```python
from build123d import *

# Parameters (mm, degrees)
BOSS_EXTRUDE1_DEPTH    = 201
CUT_EXTRUDE1_START     = -40
CUT_EXTRUDE1_OUTLINE_W = 106
CUT_EXTRUDE1_OUTLINE_H = 171
CUT_EXTRUDE1_DEPTH     = 40
SKETCH3_R              = 7.5
BOSS_EXTRUDE2_DEPTH    = 171
SKETCH4_W              = 15
SKETCH4_H              = 171
CUT_EXTRUDE2_DEPTH     = 12.5


# Read off the part's stored shape, not the designer's step: Cut-Extrude1
with BuildPart() as part:
    # Sketch1 → Boss-Extrude1 (new body)
    with BuildSketch(Plane(origin=(0, 0, 0), x_dir=(1, 0, 0), z_dir=(0, 1, 0))):
        with BuildLine():
            Line((-100, 20), (0, 20))
            ThreePointArc((0, 20), (20, 0), (0, -20))
            Line((0, -20), (-100, -20))
            Line((-100, -20), (-100, 20))
        make_face()
    extrude(amount=BOSS_EXTRUDE1_DEPTH)

    # Cut-Extrude1 outline → Cut-Extrude1 (cut)
    with BuildSketch(Plane.XY.offset(20).offset(CUT_EXTRUDE1_START)):
        with Locations((-32, 100.5)):
            Rectangle(CUT_EXTRUDE1_OUTLINE_W, CUT_EXTRUDE1_OUTLINE_H)
    extrude(amount=CUT_EXTRUDE1_DEPTH, mode=Mode.SUBTRACT)

    # Sketch3 → Boss-Extrude2 (add)
    with BuildSketch(Plane(origin=(0, 15, 0), x_dir=(1, 0, 0), z_dir=(0, 1, 0))):
        with Locations(Location((0, 0, 0), (0, 0, 90))):
            Circle(SKETCH3_R)
    extrude(amount=BOSS_EXTRUDE2_DEPTH)

    # Sketch4 → Cut-Extrude2 (cut)
    with BuildSketch(Plane.XY.offset(20)):
        with Locations((-92.5, 100.5)):
            Rectangle(SKETCH4_W, SKETCH4_H)
    extrude(amount=-CUT_EXTRUDE2_DEPTH, mode=Mode.SUBTRACT)


solid = part.part
```
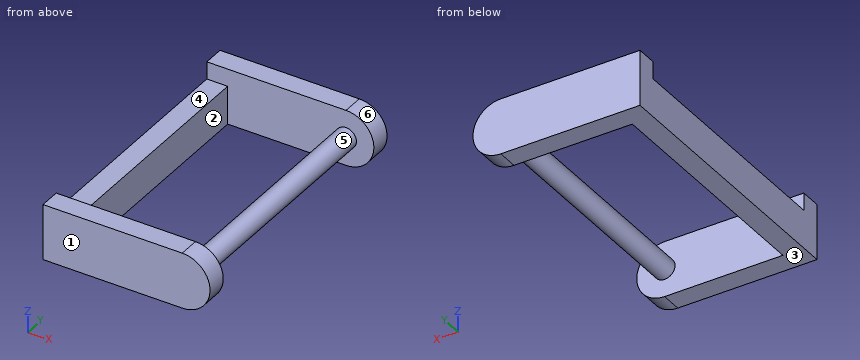
Can you work these out from the model? Positions are in its coordinate system, mm. Face numbers are marked on the shaded views. A direction names the side the tool comes from. Coordinates: 2 decimals unless noted, no trailing zeros. Write each loop counter-clockwise with the first axis right and the second up, starting at its lowest first coordinate (ties: lowest second). Pieces come first, ordered by that corner, then holes. Notation, with made-up numbers: (0, -26.75) - (54, -26.75) arc R19 cw to (54, -1.75) - close; hole circle Ø1 at (-39.5, -23). An arc over 180 degrees is marked (long way). Return JSON: item names as keys, results as strings.
Q1. I'm going to push flat-ended pins straight in: pin 1 Ø4.5 at (x, y) = (-90.5, 135.5) entering from +Z; pin 2 Ø10 at (y, z) = (87.5, 5.5) entering from +X; pin 3 Ø8 at (x, y) = (-4.5, 113) entering from -Z. Where does each tip first touch, or does it pass through?
Computed values:
{"pin 1": "stops at z = 7.5", "pin 2": "stops at x = 7.48", "pin 3": "stops at z = -7.48"}
Q2. If we section it at D-D (y = 177.5): Please give me the cut outline in (x, z), then the cut area to 3 significant figures.
Computed values:
{"outline": "(-100, -20) - (-85, -20) - (-85, 7.5) - (-100, 7.5) - close; circle Ø15 at (0, 0)", "area": "589 mm2"}
Q3. Thinking about a two-plate mould opening in Y: for the marked faces 1, 2 and 3, which applies, +Y half, -Y half, draft (parallel to the pull), parting line (faces both ways), or undercut?
Computed values:
{"face 1": "-Y half", "face 2": "undercut", "face 3": "draft"}
Q4. If we section it at B-B (z = 0): Please give me the cut outline in (x, y).
Computed values:
{"outline": "(-100, 0) - (20, 0) - (20, 15) - (7.5, 15) - (7.5, 186) - (20, 186) - (20, 201) - (-100, 201) - close; hole (-85, 15) - (-7.5, 15) - (-7.5, 186) - (-85, 186) - close"}
Q5. If we section it at A-A (z = 12): Please give me the cut outline in (x, y), then the cut area to 3 significant figures.
Computed values:
{"outline": "(-100, 0) - (16, 0) - (16, 15) - (-100, 15) - close; (-100, 186) - (16, 186) - (16, 201) - (-100, 201) - close", "area": "3,480 mm2"}
Q6. If we section it at C-C (x = -59.5): Please give me the cut outline in (y, z), then the cut area to 3 significant figures.
Computed values:
{"outline": "(0, -20) - (15, -20) - (15, 20) - (0, 20) - close; (186, -20) - (201, -20) - (201, 20) - (186, 20) - close", "area": "1,200 mm2"}
Q7. On a 3-axis mill with a long thin cutter (end or side, diameter ignored), from which of +Z, -Z, +X, -X, +Y, -Y can I reach the whole of each face in a straight line? I mean the marked faces 4, 5 and 6. Say none if no direction works.
Computed values:
{"face 4": "+Z, +X, -X", "face 5": "none", "face 6": "+X, +Y, -Y"}
Q8. Please list where these lines run through material, in increasing order: L1, parallel to Y at x = -14, z = 12; L2, parallel to X at y = 168, z = -5.5; L3, parallel to X at y = 44, z = -2. Write a range as from..to.
Computed values:
{"L1": "y = 0..15, 186..201", "L2": "x = -100..-85, -5.1..5.1", "L3": "x = -100..-85, -7.23..7.23"}
